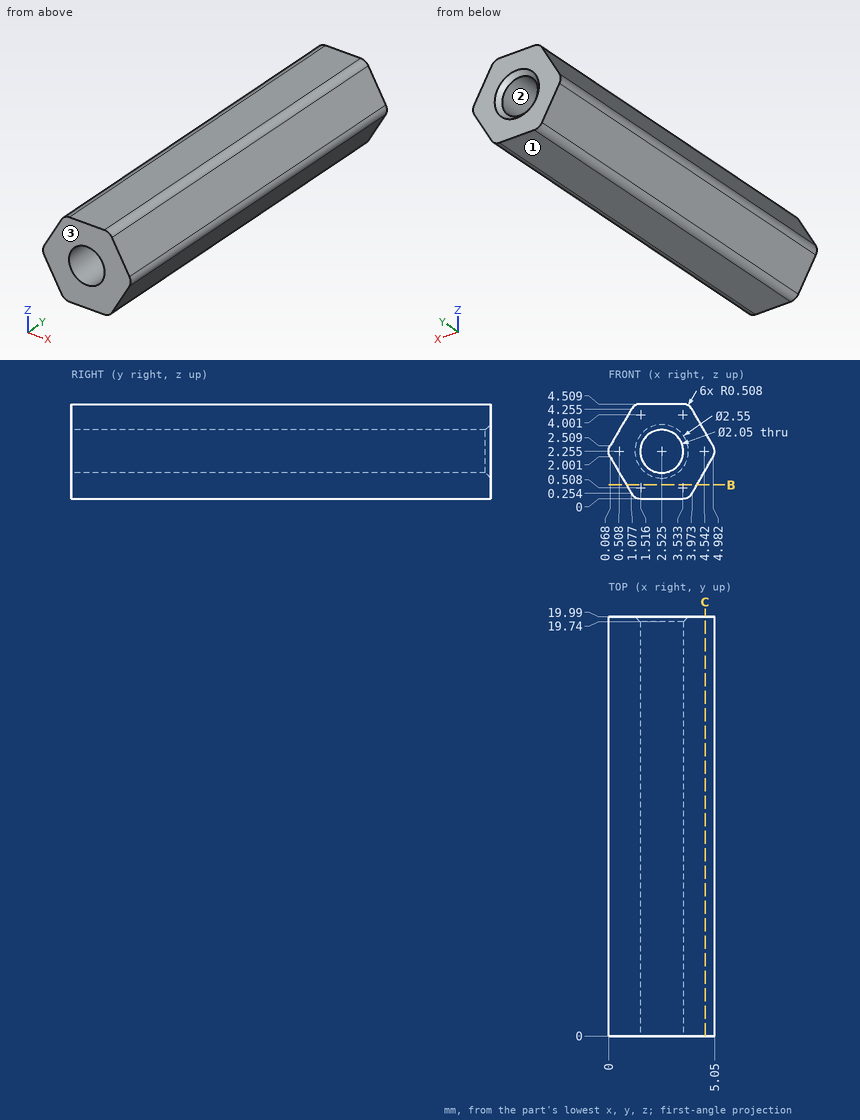
Geometry check sheet. Reference: drawing and pictorial views, mm from the part's lowest x, y, z. Coordinates: 2 decimals unless noted, no trailing zeros. Loops run counter-clockwise (first coordinate to the right, second up) from the corner with the lowest first, then second, coordinate; pieces in that order, holes last.
1) Sectioned sample at B-B (z = 0.65). Record the boundary of the cut face in (x, y).
2) Gauge pin test, flat ends, axial feed: pin 1 (1.5 mm diameter, centred on y = 8.5, z = 3.5, fed in from -X); pin 2 (1.8 mm diameter, centred on x = 2.52, z = 2.25, fed in from -Y). Record the tip position at first contact, or that the pin passes through.
3) Sectioned sample at C-C (x = 4.6). Record the boundary of the cut face in (y, z).
4) Release check for a two-part mould opening along Z. For the marked faces 1, 2 and 3 record: released by +Z, released by -Z, zero draft, split by the parting line, or undercut.
5) Material ranges on probe 1 along X at (y, z) = (14.5, 2.1) (1 decimal); probe 2 along X at (y, z) = (19, 2.9) (1 decimal); probe 3 along Z at (x, y) = (2.95, 2.25), recorded low to high.
Check sheet entries:
1. outline: (0.85, 0) - (4.2, 0) - (4.2, 19.99) - (0.85, 19.99) - close
2. pin 1: stops at x = 0.21
2. pin 2: passes through
3. outline: (0, 1.34) - (19.99, 1.34) - (19.99, 3.17) - (0, 3.17) - close
4. face 1: released by -Z
4. face 2: undercut
4. face 3: zero draft
5. probe 1: x = 0 to 1.5, 3.5 to 5
5. probe 2: x = 0.3 to 1.7, 3.3 to 4.8
5. probe 3: z = 0 to 1.32, 3.19 to 4.51
